Autodesk Inventor part; units mm, degrees
ref_plane "YZ Plane" through (0, 0, 0) normal (1, 0, 0) x (0, 1, 0)
ref_plane "XZ Plane" through (0, 0, 0) normal (0, 1, 0) x (-1, 0, 0)
ref_plane "XY Plane" through (0, 0, 0) normal (0, 0, 1) x (1, 0, 0)
sketch "Sketch1" plane through (0, 0, 0) normal (0, 0, 1) x (1, 0, 0)
  line L0 (-13.6697, 534.1801) -> (367.3303, 534.1801)
  line L1 (367.3303, 534.1801) -> (367.3303, -10.1056)
  line L2 (367.3303, -10.1056) -> (-13.6697, -10.1056)
  line L3 (-13.6697, -10.1056) -> (-13.6697, 534.1801)
  point P0 (0, 0)
  dimension "d0" = 381
  dimension "d1" = 544.2857
extrude "Extrusion1" add sketch "Sketch1" along normal blind 163.2857
sketch "Sketch2" plane through (-13.6697, 534.1801, 0) normal (0, 1, 0) x (1, 0, 0)
  line L0 (27.2143, -136.0717) -> (353.786, -136.0717)
  line L1 (353.786, -136.0717) -> (353.786, -27.214)
  line L2 (353.786, -27.214) -> (27.2143, -27.214)
  line L3 (27.2143, -27.214) -> (27.2143, -136.0717)
  line L4 (0, 0) -> (0, -163.2857)
  line L5 (381, 0) -> (0, 0)
  line L6 (381, 0) -> (381, -163.2857)
  line L7 (381, -163.2857) -> (0, -163.2857)
  point P0 (13.6697, 0)
  dimension "d4" = 27.2143
  dimension "d5" = 27.214
  dimension "d6" = 27.214
  dimension "d7" = 27.214
extrude "Extrusion2" cut sketch "Sketch2" against normal blind 218.3674 contours L3 L2 L1 L0
sketch "Sketch3" plane through (-13.6697, 315.8127, 0) normal (0, 1, 0) x (1, 0, 0)
  line L0 (353.786, -27.214) -> (353.786, -136.0717)
  line L1 (27.2143, -27.214) -> (353.786, -27.214)
  line L2 (353.786, -136.0717) -> (209.768, -136.0717)
  line L3 (209.768, -136.0717) -> (209.768, -27.214)
  line L4 (209.768, -27.214) -> (353.786, -27.214)
  line L5 (353.786, -27.214) -> (353.786, -136.0717)
  line L6 (353.786, -136.0717) -> (27.2143, -136.0717)
  line L7 (27.2143, -136.0717) -> (171.2323, -136.0717)
  line L8 (171.2323, -136.0717) -> (171.2323, -27.214)
  line L9 (171.2323, -27.214) -> (27.2143, -27.214)
  line L10 (27.2143, -27.214) -> (27.2143, -136.0717)
  point P0 (13.6697, 0)
  point P1 (27.2143, -27.214)
  point P2 (171.2323, -27.214)
  dimension "d10" = 144.018
  dimension "d11" = 144.018
extrude "Extrusion3" cut sketch "Sketch3" against normal blind 436.0817 contours L0 L2 L3 L1 | L8 L6 L10 L1
sketch "Sketch4" plane through (-13.6697, 315.8127, 0) normal (0, 1, 0) x (1, 0, 0)
  line L0 (171.2323, -27.214) -> (209.768, -27.214)
  line L1 (209.768, -136.0717) -> (209.768, -27.214)
  line L2 (171.2323, -27.214) -> (209.768, -27.214)
  line L3 (209.768, -27.214) -> (209.768, -136.0717)
  line L4 (209.768, -136.0717) -> (171.2323, -136.0717)
  line L5 (171.2323, -136.0717) -> (171.2323, -27.214)
  point P0 (13.6697, 0)
extrude "Extrusion4" cut sketch "Sketch4" against normal blind 54.4286
sketch "Sketch5" plane through (13.5445, 534.1801, 27.214) normal (0, 0, 1) x (1, 0, 0)
  line L0 (144.018, -272.796) -> (182.5537, -272.796)
  line L1 (163.2859, -272.796) -> (163.2859, -37.2995) construction
  circle A0 centre (163.2859, -251.0246) radius 13.6071
  point P0 (-13.5445, -534.1801)
  dimension "d16" = 27.2143
  dimension "d17" = 21.7714
extrude "Extrusion5" cut sketch "Sketch5" along normal mid plane 489.8571
sketch "Sketch6" plane through (-13.6697, 534.1801, 0) normal (0, 1, 0) x (1, 0, 0)
  line L0 (381, -163.2857) -> (0, -163.2857)
  line L1 (0, 0) -> (0, -163.2857)
  line L2 (27.2143, -163.2857) -> (0, -163.2857)
  line L3 (0, -163.2857) -> (0, 0)
  line L4 (0, 0) -> (26.8469, 0)
  line L5 (27.2143, -27.214) -> (27.2143, -163.2857)
  line L6 (27.2143, -27.214) -> (353.786, -27.214)
  line L7 (381, 0) -> (381, -163.2857)
  line L8 (27.2143, -27.214) -> (353.786, -27.214)
  line L9 (381, -27.214) -> (381, 0)
  line L10 (381, 0) -> (27.2143, 0)
  line L11 (381, 0) -> (0, 0)
  line L12 (381, -163.2857) -> (353.786, -163.2857)
  line L13 (353.786, -163.2857) -> (353.786, -27.214)
  line L14 (353.786, 0) -> (381, 0)
  line L15 (381, 0) -> (381, -163.2857)
  line L16 (27.2143, -27.214) -> (27.2143, -136.0717)
  line L17 (27.2143, -163.2857) -> (27.2143, -27.214)
  line L18 (27.2143, -27.214) -> (353.786, -27.214)
  line L19 (353.786, -136.0717) -> (353.786, -27.214)
  line L20 (353.786, -27.214) -> (353.786, -163.2857)
  point P0 (13.6697, 0)
extrude "Extrusion6" add sketch "Sketch6" along normal blind 304.8 contours L0 L13 L6 L5 L1 L4 L11 L10 L7
sketch "Sketch7" plane through (13.5445, -10.1056, 27.214) normal (0, 0, 1) x (1, 0, 0)
  line L0 (-27.2143, 849.0857) -> (0, 849.0857)
  line L1 (326.5717, 849.0857) -> (326.5717, 0)
  line L2 (0, 849.0857) -> (326.5717, 849.0857)
  line L3 (326.5717, 849.0857) -> (326.5717, 805.1588)
  line L4 (326.5717, 805.1588) -> (0, 805.1588)
  line L5 (0, 805.1588) -> (0, 849.0857)
  point P0 (-13.5445, 10.1056)
extrude "Extrusion7" add sketch "Sketch7" along normal up to surface (136.0717 mm away)
sketch "Sketch8" plane through (13.5445, 534.1801, 163.2857) normal (0, 1, 0) x (1, 0, 0)
  line L0 (0, 27.214) -> (144.018, 27.214)
  line L1 (0, 27.214) -> (353.7857, 27.214)
  line L2 (353.7857, 27.214) -> (353.7857, 0)
  line L3 (353.7857, 0) -> (0, 0)
  line L4 (0, 0) -> (0, 27.214)
  point P0 (-13.5445, 163.2857)
  point P1 (144.018, 27.214)
extrude "Extrusion8" add sketch "Sketch8" along normal blind 300
sketch "Sketch9" plane through (0, 0, 0) normal (0, 0, -1) x (-1, 0, 0)
  line L0 (-340.3303, 794.9801) -> (-13.3303, 794.9801)
  line L1 (-13.3303, 794.9801) -> (-13.3303, 627.4847)
  line L2 (-340.3303, 794.9801) -> (-340.3303, 627.4847)
  line L3 (-340.3303, 627.4847) -> (-13.3303, 627.4847)
  line L4 (-367.3303, 838.9801) -> (13.6697, 838.9801)
  line L5 (13.6697, -10.1056) -> (13.6697, 838.9801)
  line L6 (-367.3303, -10.1056) -> (-367.3303, 838.9801)
  point P0 (0, 0)
  dimension "d26" = 44
  dimension "d27" = 27
  dimension "d28" = 27
extrude "Extrusion9" cut sketch "Sketch9" against normal blind 50
sketch "Sketch10" plane through (0, 0, 0) normal (0, 0, -1) x (-1, 0, 0)
  point P0 (0, 0)
sketch "Sketch11" plane through (340.3303, 627.4847, 0) normal (-1, 0, 0) x (0, 0, 1)
  point P0 (0, -627.4847)
sketch "Sketch12" plane through (0, 0, 163.2857) normal (0, 0, 1) x (1, 0, 0)
  circle A0 centre (176.8304, 283.1555) radius 13.6071
  line L0 (194.8304, 297.5763) -> (176.8304, 297.5763)
  line L1 (194.8304, 297.5763) -> (199.5304, 297.5763)
  line L2 (199.5304, 297.5763) -> (199.5304, 268.7347)
  line L3 (176.8304, 297.5763) -> (152.6961, 297.5763)
  line L4 (152.6961, 297.5763) -> (152.6961, 289.0555)
  line L5 (176.8304, 283.1555) -> (176.8304, 289.0555) construction
  line L6 (176.8304, 289.0555) -> (193.4304, 289.0555)
  line L7 (193.4304, 289.0555) -> (193.4304, 285.8555)
  line L8 (176.8304, 289.0555) -> (152.6961, 289.0555)
  line L9 (176.8304, 283.1555) -> (183.0707, 283.1555) construction
  line L10 (194.8304, 268.7347) -> (176.8304, 268.7347)
  line L11 (176.8304, 268.7347) -> (152.6961, 268.7347)
  line L12 (152.6961, 268.7347) -> (152.6961, 277.2555)
  line L13 (176.8304, 277.2555) -> (193.4304, 277.2555)
  line L14 (176.8304, 277.2555) -> (152.6961, 277.2555)
  line L15 (194.8304, 268.7347) -> (199.5304, 268.7347)
  line L16 (193.4304, 277.2555) -> (193.4304, 285.8555)
  point P0 (0, 0)
  dimension "d35" = 5.9
extrude "Extrusion10" add sketch "Sketch12" along normal blind 8.3 contours L6 L8 A0 | A0 L8 L4 L3 L0 L1 L2 L15 L10 L11 L12 L14 L13 L16 L7 L6 | A0 L14 L13
properties part number "ENGR131 KC Design 2"
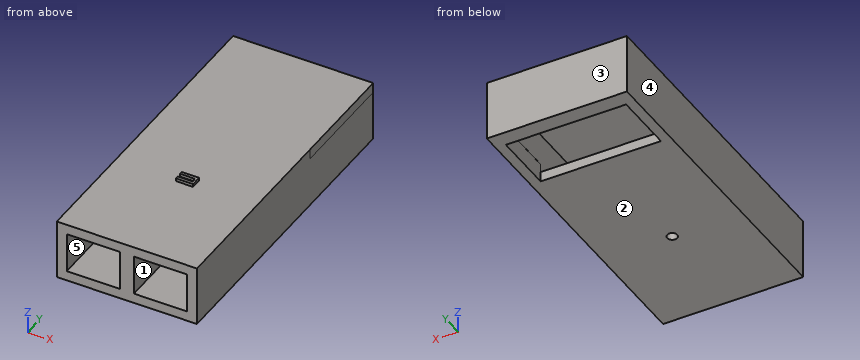
Here's how the part is built. I have some questions about the finished solid (model axes, mm). Face numbers are marked on the shaded views. A direction names the side the tool comes from. Coordinates: 2 decimals unless noted, no trailing zeros. Order: outer loops, then holes, each group sorted by start corner. A loop starts at its lowest first (then second) coordinate and runs counter-clockwise, first axis right, second up. Notation, with made-up numbers: (77.5, 54.25) - (125.5, 54.25) arc R21 cw to (125.5, 84.25) - close; hole circle Ø10 at (-37.5, -13). An arc over 180 degrees is marked (long way). One line per question, with ' | ' between items. Start each with the question number.
1. If we section it at C-C (x = 63): Write out the boundary of the cut face in (y, z).
2. I'm going to push flat-ended pins straight in: pin 1 Ø9 at (x, z) = (175, 169) entering from -Y; pin 2 Ø4 at (x, z) = (133.5, 108) entering from -Y; pin 3 Ø2.5 at (x, z) = (172, 166) entering from +Y. Where does each tip first touch, or does it pass through?
3. Which directions (+Z, -Z, +X, -X, +Y, -Y) give clear straight access to the entire face, cutting with the end or side of a thin tool? Please do the marked faces 1 and 2.
4. Please list where these lines run through material, in increasing order: line 1 along X through (y, z) = (105.5, 93); line 2 along Z through (x, y) = (286.5, 587.5); line 3 along Y through (x, z) = (161.5, 45). Write a range as [from, to].
5. If we section it at D-D (y = 108): Write out the boundary of the cut face in (x, z), and give its area (3 significant figures).
6. If we section it at A-A (z = 62.5): Write out the boundary of the cut face in (x, y).
7. If we section it at B-B (y = 471.5): Write out the boundary of the cut face in (x, z).
8. If we mould it in two halves opening along X, with no side actions, what happens to the marked faces 3, 4 and 5? For each: released by +X, released by -X, zero draft, split by the parting line, or undercut.
Model answer:
1) outline: (-10.11, 0) - (627.48, 0) - (627.48, 27.21) - (-10.11, 27.21) - close; (-10.11, 136.07) - (795.05, 136.07) - (795.05, 27.21) - (794.98, 27.21) - (794.98, 0) - (838.98, 0) - (838.98, 163.29) - (-10.11, 163.29) - close
2) pin 1: stops at y = 268.73 | pin 2: stops at y = 795.05 | pin 3: stops at y = 297.58
3) face 1: -Y | face 2: -Z, +X, -X, +Y, -Y
4) line 1: x = [-13.67, 13.54], [157.56, 196.1], [340.12, 367.33] | line 2: z = [0, 27.21], [136.07, 163.29] | line 3: y = [-10.11, 261.38], [795.05, 838.98]
5) outline: (-13.67, 0) - (367.33, 0) - (367.33, 163.29) - (-13.67, 163.29) - close; hole (13.54, 27.21) - (157.56, 27.21) - (157.56, 136.07) - (13.54, 136.07) - close; hole (196.1, 27.21) - (340.12, 27.21) - (340.12, 136.07) - (196.1, 136.07) - close | area: 30,900 mm²
6) outline: (-13.67, -10.11) - (13.54, -10.11) - (13.54, 795.05) - (340.12, 795.05) - (340.12, -10.11) - (367.33, -10.11) - (367.33, 838.98) - (-13.67, 838.98) - close; (157.56, -10.11) - (196.1, -10.11) - (196.1, 261.38) - (157.56, 261.38) - close
7) outline: (-13.67, 0) - (367.33, 0) - (367.33, 163.29) - (-13.67, 163.29) - close; hole (13.54, 27.21) - (340.12, 27.21) - (340.12, 136.07) - (13.54, 136.07) - close
8) face 3: zero draft | face 4: released by -X | face 5: undercut
